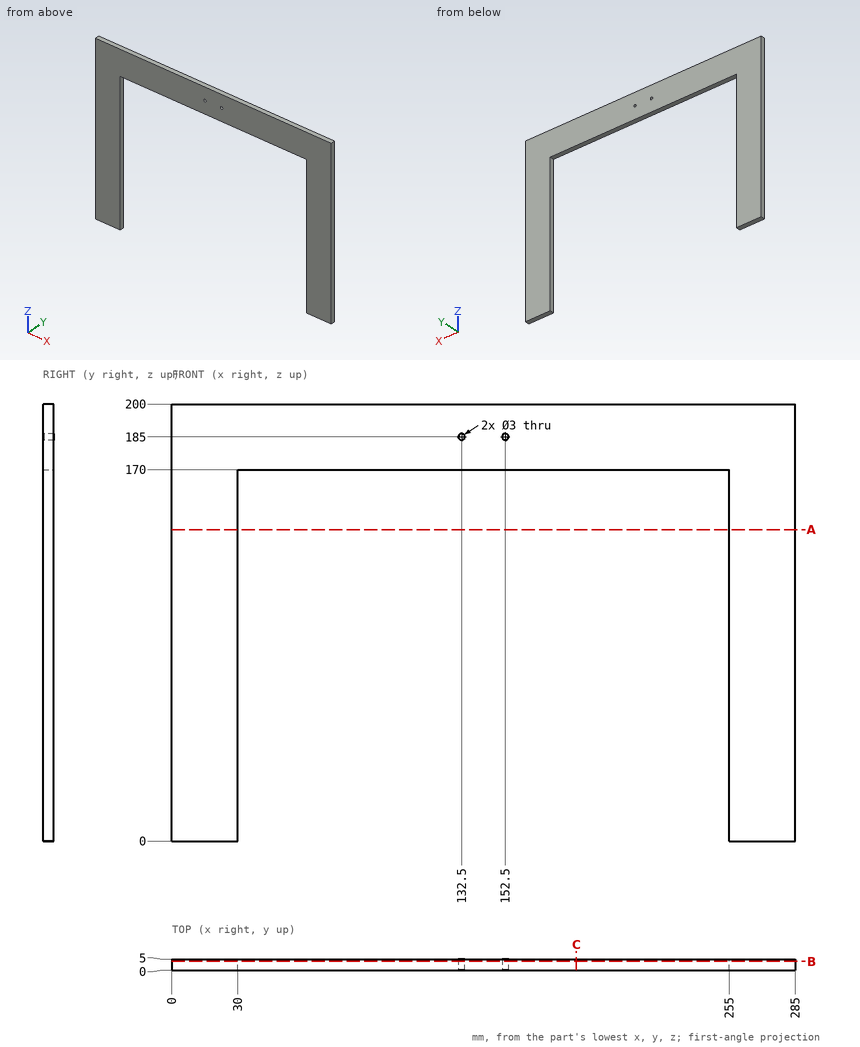
Study the drawing (mm; zero at the part's minimum x, y, z) and answer. Give positions to 0.01 mm unless a question says otherwise; leave off trailing zeros. Loops run counter-clockwise (first coordinate to the right, second up) from the corner with the lowest first, then second, coordinate; pieces in that order, holes last. Notation, with made-up numbers: (-26.5, 72) - (-15.5, 72) arc R17 cw to (-15.5, 77) - close; hole circle Ø9 at (16.5, 5). An arc over 180 degrees is marked (long way). Answer in a Markdown table with one row per item. Add a question column.
Q1. Consider line 1 along X through (y, z) = (1.25, 185); line 2 along Z through (x, y) = (152.5, 3.7); line 3 along X through (y, z) = (3.45, 36). Determine where each line is inside the solid, lowest interval first.
Q2. The part is cut by section B-B (y = 4). Determine the outline of the cut face in (x, z).
Q3. Each of these flat-tipped pins is pushed along its axis until it touches: P1, Ø2.5, axis at x = 180, y = 3.5, coming from the -Z side; P2, Ø2.5, axis at x = 152.5, z = 185, coming from the -Y side. Where does it stop, or does it pass through?
Q4. The part is cut by section A-A (z = 142.5). Determine the outline of the cut face in (x, y).
Q5. The part is cut by section C-C (x = 185). Determine the outline of the cut face in (y, z).
Solution:
| question | item | result |
|---|---|---|
| 1 | line 1 | x = 0 to 131, 134 to 151, 154 to 285 |
| 1 | line 2 | z = 170 to 183.5, 186.5 to 200 |
| 1 | line 3 | x = 0 to 30, 255 to 285 |
| 2 | outline | (0, 0) - (30, 0) - (30, 170) - (255, 170) - (255, 0) - (285, 0) - (285, 200) - (0, 200) - close; hole circle Ø3 at (132.5, 185); hole circle Ø3 at (152.5, 185) |
| 3 | P1 | stops at z = 170 |
| 3 | P2 | passes through |
| 4 | outline | (0, 0) - (30, 0) - (30, 5) - (0, 5) - close; (255, 0) - (285, 0) - (285, 5) - (255, 5) - close |
| 5 | outline | (0, 170) - (5, 170) - (5, 200) - (0, 200) - close |
